Source: CAD feature listing. Evaluate the final solid. Frame: model axes, mm. A direction names the side the tool comes from. Give positions to 0.01 mm unless a question says otherwise; leave off trailing zeros. Loops run counter-clockwise (first coordinate to the right, second up) from the corner with the lowest first, then second, coordinate; pieces in that order, holes last. Notation, with made-up numbers: (28.5, 68.5) -> (73.5, 68.5) arc R20 cw to (73.5, 106.5) -> close; hole circle Ø2 at (11, 0.5). An arc over 180 degrees is marked (long way). Return JSON: item names as keys, results as strings. Group by question number.
(1) Pin query (flat end, axial travel): pin 1 (0.5 mm diameter, centred on y = -14.5, z = 10.5, fed in from +X); pin 2 (11 mm diameter, centred on x = -12, z = -3.5, fed in from +Y); pin 3 (2.5 mm diameter, centred on x = -0.5, z = 0, fed in from +Y). Return the tip coordinate at first contact, or that it passes through.
(2) Cut plane C-C on y = -5.5. Return loops of the section in (x, z), then the cut area to 3 significant figures.
(3) Cut plane A-A on x = 7. Return loops of the section in (y, z), then the cut area to 3 significant figures.
(4) Cut plane D-D on x = 18.5. Return loops of the section in (y, z), then the cut area to 3 significant figures.
(5) Ray query, line 1 (Z direction, x = 0, y = -13.25); line 2 (Z direction, x = 3, y = -12.5); line 3 (Y direction, x = 19, z = -5.5). Return the intervals inside material, ascending. Write a range as from..to.
(6) Draft query along Y for faces 1 (the face through (2, 0, -2)), 2 (the face through (0, -14, 10)), 3 (the face through (0, -14, -11)), 4 (the face through (15, -14.5, 10.5)). Return one class per face: released by +Y, released by -Y, zero draft, split by the parting line, or undercut.
(7) Cut plane B-B on z = 0. Return loops of the section in (x, y).
(8) Access query for faces 5 (the face through (15, -14.5, -10.5)), 6 (the face through (-0.59, -4.93, 4.46)), 7 (the face through (0, -12, 5)), 8 (the face through (-15, -14.5, 10.5)). Directions: +Z, -Z, +X, -X, +Y, -Y. A direction counts if a zero-diameter tool reaches every point of the face in a straight line with its end or side. Return the directions, or none.
```python
from build123d import *

# Parameters (mm, degrees)
SKETCH_R      = 4.5
SKETCH_R_2    = 2.5
PAD_DEPTH     = 10
SKETCH001_R   = 2.5
PAD001_DEPTH  = 2
SKETCH002_R   = 4.5
SKETCH002_R_2 = 2.5
SKETCH002_W   = 30
SKETCH002_H   = 1
PAD002_DEPTH  = 5
PAD003_DEPTH  = 2


with BuildPart() as part:
    # Sketch → Pad (new body)
    with BuildSketch(Plane.XZ):
        Circle(SKETCH_R)
        Circle(SKETCH_R_2, mode=Mode.SUBTRACT)
    extrude(amount=PAD_DEPTH)

    # Sketch001 → Pad001 (new body)
    with BuildSketch(Plane.XZ.offset(10)):
        with BuildLine():
            Line((15.499965, -11), (-15.499965, -11))
            ThreePointArc((-15.499965, 11), (-26.5, 0), (-15.499965, -11))
            Line((-15.499965, 11), (15.499965, 11))
            ThreePointArc((15.499965, -11), (26.5, 0), (15.499965, 11))
        make_face()
        Circle(SKETCH001_R, mode=Mode.SUBTRACT)
    extrude(amount=PAD001_DEPTH)

    # Sketch002 → Pad002 (new body)
    with BuildSketch(Plane.XZ.offset(12)):
        Circle(SKETCH002_R)
        Circle(SKETCH002_R_2, mode=Mode.SUBTRACT)
        with Locations((0, 10.5)):
            Rectangle(SKETCH002_W, SKETCH002_H)
        with Locations((0, -10.5)):
            Rectangle(SKETCH002_W, SKETCH002_H)
    extrude(amount=PAD002_DEPTH)

    # Sketch003 → Pad003 (new body)
    with BuildSketch(Plane.XZ.offset(17)):
        with BuildLine():
            Line((-15.5, 11), (15.5, 11))
            ThreePointArc((15.499965, -11), (26.499965, -1.7e-05), (15.5, 11))
            Line((15.499965, -11), (-15.499963, -11))
            ThreePointArc((-15.5, 11), (-26.499965, -1.8e-05), (-15.499963, -11))
        make_face()
    extrude(amount=PAD003_DEPTH)


solid = part.part
```
Answers:
{
 "1": {"pin 1": "x = 15", "pin 2": "y = -10", "pin 3": "y = -17"},
 "2": {"outline": "circle Ø9 at (0, 0); hole circle Ø5 at (0, 0)", "area": "44.0 mm²"},
 "3": {"outline": "(-19, -11) -> (-10, -11) -> (-10, 11) -> (-19, 11) -> close; hole (-17, -10) -> (-12, -10) -> (-12, 10) -> (-17, 10) -> close", "area": "98.0 mm²"},
 "4": {"outline": "(-19, -10.58) -> (-17, -10.58) -> (-17, 10.58) -> (-19, 10.58) -> close; (-12, -10.58) -> (-10, -10.58) -> (-10, 10.58) -> (-12, 10.58) -> close", "area": "84.7 mm²"},
 "5": {"line 1": "-11..-10, -4.5..-2.5, 2.5..4.5, 10..11", "line 2": "-11..-10, -3.35..3.35, 10..11", "line 3": "-19..-17, -12..-10"},
 "6": {"face 1": "released by +Y", "face 2": "undercut", "face 3": "zero draft", "face 4": "undercut"},
 "7": {"outline": "(-26.5, -19) -> (26.5, -19) -> (26.5, -17) -> (4.5, -17) -> (4.5, -12) -> (26.5, -12) -> (26.5, -10) -> (4.5, -10) -> (4.5, 0) -> (2.5, 0) -> (2.5, -17) -> (-2.5, -17) -> (-2.5, 0) -> (-4.5, 0) -> (-4.5, -10) -> (-26.5, -10) -> (-26.5, -12) -> (-4.5, -12) -> (-4.5, -17) -> (-26.5, -17) -> close"},
 "8": {"face 5": "+Z, -Z, +X", "face 6": "+Y", "face 7": "none", "face 8": "+Z, -Z, -X"}
}
